Design review of the part built by this model. Coordinates are the model's own, in mm. Face numbers are marked on the shaded views. A direction names the side the tool comes from. Coordinates: 2 decimals unless noted, no trailing zeros. Loops run counter-clockwise (first coordinate to the right, second up) from the corner with the lowest first, then second, coordinate; pieces in that order, holes last. Notation, with made-up numbers: (26.25, 84.25) -> (35.25, 84.25) arc R27 ccw to (35.25, 116.25) -> close; hole circle Ø7 at (-40, 36). An arc over 180 degrees is marked (long way). Answer in a Markdown table with one row per item.
```python
from build123d import *

# Parameters (mm, degrees)
F0_W     = 15
F0_H     = 47
F0_R     = 11.35
F1_DEPTH = 3.5
F2_DEPTH = 15
F3_T     = -3
F4_R     = 2.5
F5_DEPTH = 56


# Not quite as in the source:
# - a shell that OpenCascade refuses in one call is made with other operations: the cavity is built on its own and cut out


with BuildPart() as f1:
    # F0 (on Front) → F1 (new body, symmetric)
    with BuildSketch(Plane.XZ):
        with Locations((7.5, -23.5)):
            Rectangle(F0_W, F0_H)
        with BuildLine():
            Line((0, 0), (15, 0))
            Line((15, 0), (15, 34.5828086023))
            ThreePointArc((15, 34.5828086023), (10.6066017178, 23.9762068845), (0, 19.5828086023))
            Line((0, 19.5828086023), (0, 0))
        make_face()
        with BuildLine():
            ThreePointArc((15, 34.5828086023), (0, 49.5828086023), (-15, 34.5828086023))
            ThreePointArc((-15, 34.5828086023), (-10.6066017178, 23.9762068845), (0, 19.5828086023))
            ThreePointArc((0, 19.5828086023), (10.6066017178, 23.9762068845), (15, 34.5828086023))
        make_face()
        with Locations((0, 34.5828086023)):
            Circle(F0_R, mode=Mode.SUBTRACT)
        with BuildLine():
            Line((-15, 34.5828086023), (-15, 0))
            Line((-15, 0), (0, 0))
            Line((0, 0), (0, 19.5828086023))
            ThreePointArc((0, 19.5828086023), (-10.6066017178, 23.9762068845), (-15, 34.5828086023))
        make_face()
        with Locations((-7.5, -23.5)):
            Rectangle(F0_W, F0_H)
    extrude(amount=F1_DEPTH, both=True)

    # F0 (on Front) → F2 (join, symmetric)
    with BuildSketch(Plane.XZ):
        Polygon((-25, -47), (-25, -50), (25, -50), (25, -47), (15, -47), (0, -47), (-15, -47), align=None)
    extrude(amount=F2_DEPTH, both=True)

    # F3: a shell. OpenCascade refuses it in one call, so the cavity is built on its own and cut out:
    # the body offset inwards by the wall thickness, plus a prism from it out through each open face.
    f3_core = offset(f1.part, amount=F3_T, kind=Kind.INTERSECTION, mode=Mode.PRIVATE)
    f3_exits = [f3_core.faces().sort_by_distance(p)[0] for p in [
        (0, 0.5, -12.400343),
    ]]
    add(f3_core, mode=Mode.SUBTRACT)
    extrude(f3_exits, amount=-F3_T, mode=Mode.SUBTRACT)

    # F4 (on Top) → F5 (cut)
    with BuildSketch(Plane.XY):
        with Locations((20, 10)):
            Circle(F4_R)
        with Locations((-20, 10)):
            Circle(F4_R)
        with Locations((-20, -10)):
            Circle(F4_R)
        with Locations((20, -10)):
            Circle(F4_R)
    extrude(amount=-F5_DEPTH, mode=Mode.SUBTRACT)


solid = f1.part
```
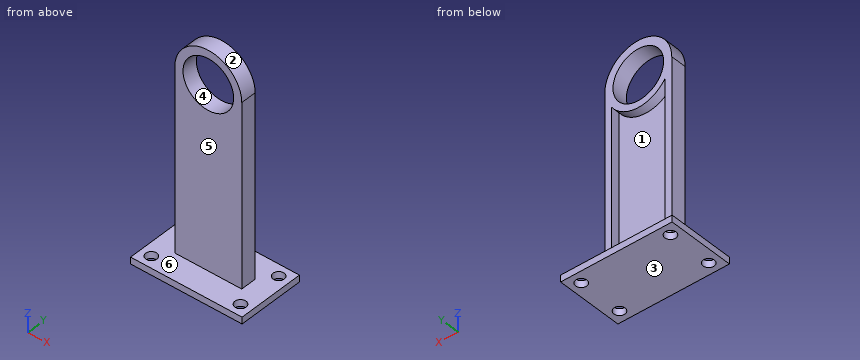
(1) Draft analysis for pull direction X (two halves, no side actions). For the marked faces 1, 2 and 3, state which applies: pulls with the +X half, pulls with the -X half, needs draft (parallel to the pull), parting line crosses it, or undercut.
Evaluation:
| item | result |
|---|---|
| face 1 | undercut |
| face 2 | parting line crosses it |
| face 3 | needs draft |
(2) For pin 1 (15 mm diameter, centred on x = -11, y = 2.5, fed in from +Z); pin 2 (6.5 mm diameter, centred on x = 20, y = -10, fed in from -Z); pin 3 (3 mm diameter, centred on y = 2.5, z = -25.5, fed in from -X); pin 4 (5 mm diameter, centred on x = 11.5, z = 10, fed in from -Y), all flat-tipped, find the tip position at first contact; note any pin that passes through.
Evaluation:
| item | result |
|---|---|
| pin 1 | stops at z = 49.17 |
| pin 2 | stops at z = -50 |
| pin 3 | stops at x = -15 |
| pin 4 | stops at y = -3.5 |
(3) To check wall thickness, follow probe 1 along Y at (x, z) = (20, -48); probe 2 along Z at (x, y) = (0, 1.75); probe 3 along Z at (x, y) = (3, 1.25). State the ranges of each line that lie inside material, in increasing order.
Evaluation:
| item | result |
|---|---|
| probe 1 | y = -15 to -12.5, -7.5 to 7.5, 12.5 to 15 |
| probe 2 | z = -50 to -47, 20.23 to 23.23, 45.93 to 49.58 |
| probe 3 | z = -50 to -47, 20.55 to 23.64, 45.53 to 49.28 |
(4) Take a section at D-D on x = -20. Give the boundary of the cut face in (y, z).
Evaluation:
| item | result |
|---|---|
| outline | (-15, -50) -> (-12.5, -50) -> (-12.5, -47) -> (-15, -47) -> close; (-7.5, -50) -> (7.5, -50) -> (7.5, -47) -> (-7.5, -47) -> close; (12.5, -50) -> (15, -50) -> (15, -47) -> (12.5, -47) -> close |
(5) Tool access review of the marked faces 4, 5 and 6: name each direction out of +Z, -Z, +X, -X, +Y, -Y from which nothing blocks a thin tool from reaching the whole face with its end or side.
Evaluation:
| item | result |
|---|---|
| face 4 | +Y, -Y |
| face 5 | +Z, +X, -X, -Y |
| face 6 | none |
(6) Take a section at B-B on x = 0. Give the boundary of the cut face in (y, z), and give its area (3 significant figures).
Evaluation:
| item | result |
|---|---|
| outline | (-15, -50) -> (15, -50) -> (15, -47) -> (-0.5, -47) -> (-0.5, 20.23) -> (3.5, 20.23) -> (3.5, 23.23) -> (-3.5, 23.23) -> (-3.5, -47) -> (-15, -47) -> close; (-3.5, 45.93) -> (3.5, 45.93) -> (3.5, 49.58) -> (-3.5, 49.58) -> close |
| area | 338 mm² |
(7) Take a section at C-C on z = 19. Give the boundary of the cut face in (x, y).
Evaluation:
| item | result |
|---|---|
| outline | (-15, -3.5) -> (15, -3.5) -> (15, 3.5) -> (12, 3.5) -> (12, -0.5) -> (-12, -0.5) -> (-12, 3.5) -> (-15, 3.5) -> close |
(8) Take a section at A-A on y = -10. Give the boundary of the cut face in (x, z), and give its area (3 significant figures).
Evaluation:
| item | result |
|---|---|
| outline | (-25, -50) -> (-22.5, -50) -> (-22.5, -47) -> (-25, -47) -> close; (-17.5, -50) -> (17.5, -50) -> (17.5, -47) -> (-17.5, -47) -> close; (22.5, -50) -> (25, -50) -> (25, -47) -> (22.5, -47) -> close |
| area | 120 mm² |
